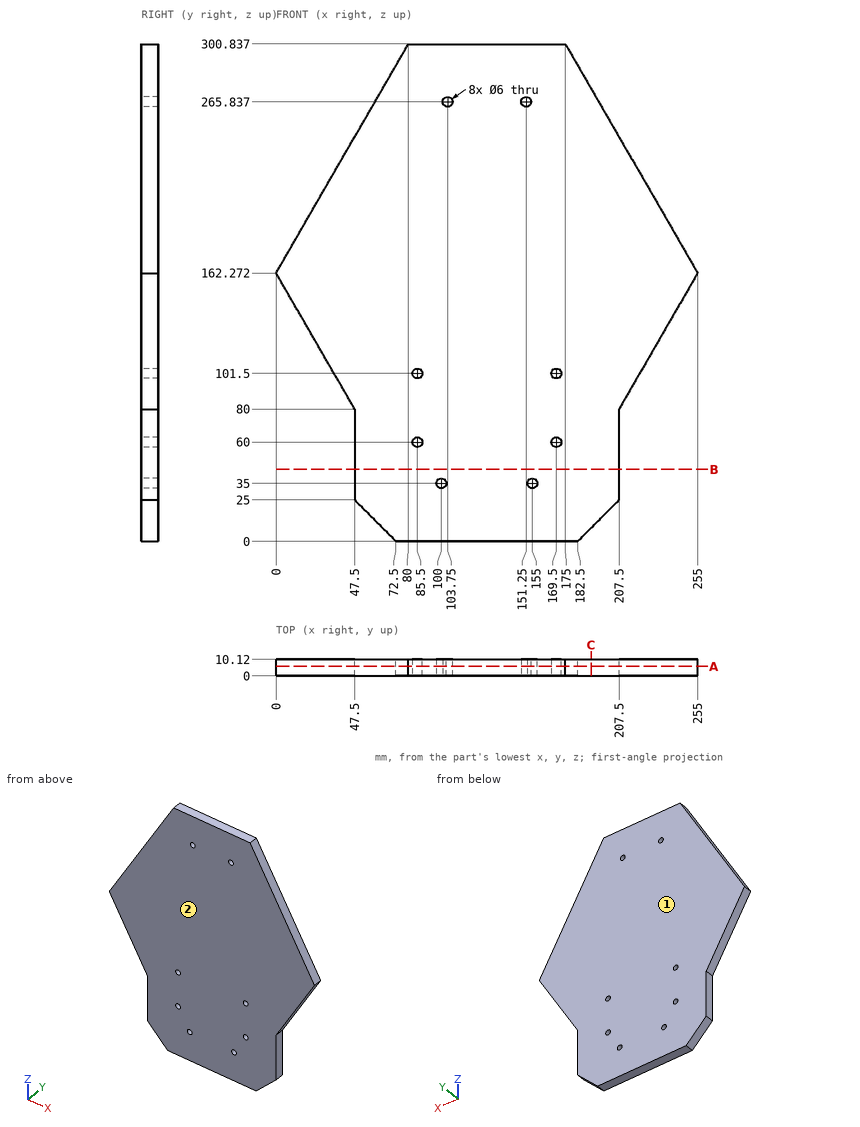
The figure shows three views and two pictorial views of one solid part (mm, origin at its lowest corner). Answer the questions. Coordinates: 2 decimals unless noted, no trailing zeros. Loops run counter-clockwise (first coordinate to the right, second up) from the corner with the lowest first, then second, coordinate; pieces in that order, holes last.
1) Find the intervals of material crossed by L1, parallel to Z at x = 169.5, y = 2; L2, parallel to X at y = 3.5, z = 35; L3, parallel to X at y = 5.75, z = 101.5 (1 decimal), in increasing order.
2) Find section C-C on x = 190.5. Write down the section's boundary in (y, z), then the cut area to 3 significant figures.
3) Flat-ended cylindrical pins translate along their axes: pin 1 Ø3 at (y, z) = (8.5, 87) entering from +X; pin 2 Ø1 at (y, z) = (4, 132.5) entering from -X; pin 3 Ø4 at (y, z) = (6.5, 162) entering from -X; pin 4 Ø5 at (y, z) = (6.5, 45) entering from -X. Find the tip coordinate at first contact, or state that the pin passes through.
4) Find section A-A on y = 5.75. Give the number of separate pieces and of enclosed holes in the cut face, then the cut area to 3 significant figures.
5) Determine the mould class of the marked faces 1 and 2 for opening direction Y: pulls with the +Y half, pulls with the -Y half, needs draft (parallel to the pull), parting line crosses it, or undercut.
6) Find section B-B on z = 43.5. Write down the section's boundary in (x, y), then the cut area to 3 significant figures.
Values:
1. L1: z = 0 to 57, 63 to 98.5, 104.5 to 300.84
1. L2: x = 47.5 to 97, 103 to 152, 158 to 207.5
1. L3: x = 35.1 to 82.5, 88.5 to 166.5, 172.5 to 219.9
2. outline: (0, 8) - (10.12, 8) - (10.12, 273.99) - (0, 273.99) - close
2. area: 2,690 mm2
3. pin 1: stops at x = 212.41
3. pin 2: stops at x = 16.9
3. pin 3: stops at x = 0
3. pin 4: stops at x = 47.5
4. separate pieces: 1
4. enclosed holes: 8
4. area: 53,300 mm2
5. face 1: pulls with the +Y half
5. face 2: pulls with the -Y half
6. outline: (47.5, 0) - (207.5, 0) - (207.5, 10.12) - (47.5, 10.12) - close
6. area: 1,620 mm2
